Geometry: final body of the model. Coordinates: model frame, mm. Face numbers are marked on the shaded views. A direction names the side the tool comes from. Give positions to 0.01 mm unless a question says otherwise; leave off trailing zeros. Loops run counter-clockwise (first coordinate to the right, second up) from the corner with the lowest first, then second, coordinate; pieces in that order, holes last.
1. Section A-A, the plane y = 0. Output: boundary loops of the cut face in (x, z) (3 decimals), then the cut area to 3 significant figures.
2. Section C-C, the plane x = -25.4. Output: boundary loops of the cut face in (y, z) (3 decimals).
3. Section B-B, the plane z = 4. State how many separate pieces and enclosed holes the cut face has, then the cut area to 3 significant figures.
4. Access query for the marked faces 1 and 2. Directions: +Z, -Z, +X, -X, +Y, -Y. A direction counts if a zero-diameter tool reaches every point of the face in a straight line with its end or side. Return the directions, or none.
5. First-contact query: P1, Ø6, axis at y = -1, z = 3, coming from the -X side; P2, Ø1.5, axis at y = 29.5, z = 1.5, coming from the -X side; P3, Ø6, axis at x = 10.5, z = 5, coming from the -Y side; P4, Ø1, axis at x = -28, z = 2, coming from the -Y side. Flat tips, straight axial feed; report the tip coordinate or a pass-through.
6. Material intervals for line 1 along X through (y, z) = (-22.5, 1); line 2 along Y through (x, z) = (-26, 2.5); line 3 along X through (y, z) = (-5.08, 3.1), sorted ascending.
from build123d import *

# Parameters (mm, degrees)
SKETCH1_R           = 31.75
BOSS_EXTRUDE1_DEPTH = 5.334
SKETCH2_R           = 38.1
BOSS_EXTRUDE2_DEPTH = 5.08
SKETCH3_R           = 3.175
CUT_EXTRUDE1_DEPTH  = 55.878697106
CIRPATTERN1_COUNT   = 4
SKETCH6_R           = 1.27
CUT_EXTRUDE3_DEPTH  = 5.334
CIRPATTERN2_COUNT   = 4


with BuildPart() as part:
    # Sketch1 → Boss-Extrude1 (new body)
    with BuildSketch(Plane.XY):
        Circle(SKETCH1_R)
    extrude(amount=BOSS_EXTRUDE1_DEPTH)

    # Sketch2 → Boss-Extrude2 (add)
    with BuildSketch(Plane.XY.offset(5.334)):
        Circle(SKETCH2_R)
    extrude(amount=BOSS_EXTRUDE2_DEPTH)

    # Sketch3 → Cut-Extrude1 (cut, through all)
    with BuildSketch(Plane.XY.offset(10.414)):
        with Locations((0, 25.4)):
            Circle(SKETCH3_R)
    cut_extrude1 = extrude(amount=-CUT_EXTRUDE1_DEPTH, mode=Mode.SUBTRACT)

    # CirPattern1: Cut-Extrude1 ×4 about axis
    cirpattern1_axis = Axis((0, 0, 0), (0, 0, 1))
    for i in range(1, CIRPATTERN1_COUNT):
        add(cut_extrude1.rotate(cirpattern1_axis, i * 360 / CIRPATTERN1_COUNT), mode=Mode.SUBTRACT)

    # Sketch6 → Cut-Extrude3 (cut)
    with BuildSketch(Plane(origin=(0, 0, 0), x_dir=(-1, 0, 0), z_dir=(0, 0, -1))):
        with Locations((-5.08, 0)):
            Circle(SKETCH6_R)
    cut_extrude3 = extrude(amount=-CUT_EXTRUDE3_DEPTH, mode=Mode.SUBTRACT)

    # CirPattern2: Cut-Extrude3 ×4 about axis
    cirpattern2_axis = Axis((0, 0, 0), (0, 0, 1))
    for i in range(1, CIRPATTERN2_COUNT):
        add(cut_extrude3.rotate(cirpattern2_axis, i * 360 / CIRPATTERN2_COUNT), mode=Mode.SUBTRACT)


solid = part.part
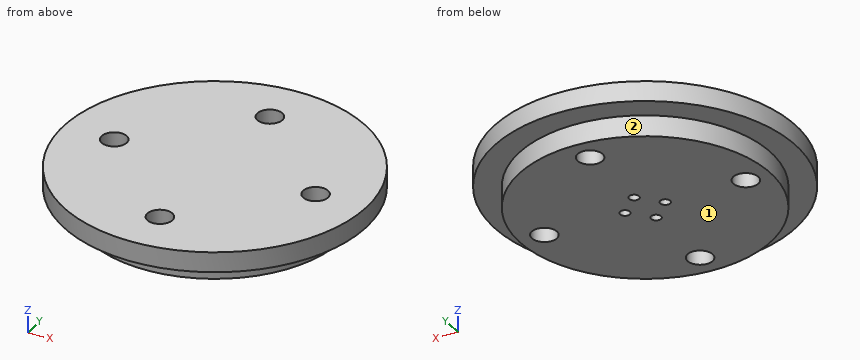
Answers below:
1. outline: (-38.1, 5.334) - (-31.75, 5.334) - (-31.75, 0) - (-28.575, 0) - (-28.575, 10.414) - (-38.1, 10.414) - close; (-22.225, 0) - (-6.35, 0) - (-6.35, 5.334) - (-3.81, 5.334) - (-3.81, 0) - (3.81, 0) - (3.81, 5.334) - (6.35, 5.334) - (6.35, 0) - (22.225, 0) - (22.225, 10.414) - (-22.225, 10.414) - close; (28.575, 0) - (31.75, 0) - (31.75, 5.334) - (38.1, 5.334) - (38.1, 10.414) - (28.575, 10.414) - close
1. area: 566 mm2
2. outline: (-28.398, 5.334) - (-19.05, 5.334) - (-19.05, 0) - (-3.175, 0) - (-3.175, 10.414) - (-28.398, 10.414) - close; (3.175, 0) - (19.05, 0) - (19.05, 5.334) - (28.398, 5.334) - (28.398, 10.414) - (3.175, 10.414) - close
3. separate pieces: 1
3. enclosed holes: 8
3. area: 3,020 mm2
4. face 1: -Z, +X, -X, +Y, -Y
4. face 2: -Z
5. P1: stops at x = -38.1
5. P2: stops at x = -13.47
5. P3: stops at y = -37.35
5. P4: stops at y = -15.87
6. line 1: x = -22.4 to -1.29, 1.29 to 22.4
6. line 2: y = -18.22 to -3.12, 3.12 to 18.22
6. line 3: x = -31.34 to -1.27, 1.27 to 31.34
